```python
from build123d import *

# Parameters (mm, degrees)
EXTRUDE_1_DEPTH               = 10
SKETCH_2_R                    = 2.5
CUT_EXTRUDE_2_DEPTH           = 39.013155617
SKETCH_4_R                    = 4.5
CUT_EXTRUDE_3_DEPTH           = 2
CUT_EXTRUDE_3_DRAFT           = -45
CUT_EXTRUDE_3_PROFILE_2_DEPTH = 2
CUT_EXTRUDE_3_PROFILE_2_DRAFT = -45
CUT_EXTRUDE_3_PROFILE_3_DEPTH = 2
CUT_EXTRUDE_3_PROFILE_3_DRAFT = -45
CUT_EXTRUDE_3_PROFILE_4_DEPTH = 2
CUT_EXTRUDE_3_PROFILE_4_DRAFT = -45
SKETCH_5_R                    = 3
CUT_EXTRUDE_4_DEPTH           = 39.013155617


with BuildPart() as part:
    # Эскиз1 → Вытянуть1 (new body)
    with BuildSketch(Plane(origin=(0, 0, 0), x_dir=(0, 0, -1), z_dir=(1, 0, 0))):
        with BuildLine():
            Line((12.845232579, 11), (33, 11))
            Line((33, 11), (33, -11))
            Line((33, -11), (12.845232579, -11))
            ThreePointArc((12.845232579, -11), (11.757018204, -11.204326651), (10.817037961, -11.789473684))
            ThreePointArc((10.817037961, -11.789473684), (0, -16), (-10.817037961, -11.789473684))
            ThreePointArc((-10.817037961, -11.789473684), (-11.757018204, -11.204326651), (-12.845232579, -11))
            Line((-12.845232579, -11), (-33, -11))
            Line((-33, -11), (-33, 11))
            Line((-33, 11), (-12.845232579, 11))
            ThreePointArc((-12.845232579, 11), (-11.757018204, 11.204326651), (-10.817037961, 11.789473684))
            ThreePointArc((-10.817037961, 11.789473684), (0, 16), (10.817037961, 11.789473684))
            ThreePointArc((10.817037961, 11.789473684), (11.757018204, 11.204326651), (12.845232579, 11))
        make_face()
    extrude(amount=EXTRUDE_1_DEPTH)

    # Эскиз2 → Вытянуть2 (cut, through all)
    with BuildSketch(Plane(origin=(10, 0, 0), x_dir=(0, 0, -1), z_dir=(1, 0, 0))):
        with Locations((0, 10)):
            Circle(SKETCH_2_R)
        with Locations((10, 0)):
            Circle(SKETCH_2_R)
        with Locations((0, -10)):
            Circle(SKETCH_2_R)
        with Locations((-10, 0)):
            Circle(SKETCH_2_R)
    extrude(amount=-CUT_EXTRUDE_2_DEPTH, mode=Mode.SUBTRACT)


with BuildPart() as cut_extrude_3_tool:
    # Эскиз4 → Вытянуть3 (with draft: the straight prism first)
    with BuildSketch(Plane(origin=(10, 0, 0), x_dir=(0, 0, -1), z_dir=(1, 0, 0))):
        with Locations((0, 10)):
            Circle(SKETCH_4_R)
    extrude(amount=-CUT_EXTRUDE_3_DEPTH)
    # Вытянуть3: the draft: its side faces are tilted about the plane it starts from
    cut_extrude_3_sides = [cut_extrude_3_tool.faces().sort_by_distance(p)[0] for p in [
        (9, 10, 4.5),
    ]]
    draft(cut_extrude_3_sides, Plane(origin=(10, 0, 0), x_dir=(0, 0, -1), z_dir=(1, 0, 0)), CUT_EXTRUDE_3_DRAFT)


with BuildPart() as part_1:
    add(part.part)

    # Вытянуть3: cut by cut_extrude_3_tool
    add(cut_extrude_3_tool.part, mode=Mode.SUBTRACT)


with BuildPart() as cut_extrude_3_profile_2_tool:
    # Эскиз4 → Вытянуть3 profile 2 (with draft: the straight prism first)
    with BuildSketch(Plane(origin=(10, 0, 0), x_dir=(0, 0, -1), z_dir=(1, 0, 0))):
        with Locations((10, 0)):
            Circle(SKETCH_4_R)
    extrude(amount=-CUT_EXTRUDE_3_PROFILE_2_DEPTH)
    # Вытянуть3 profile 2: the draft: its side faces are tilted about the plane it starts from
    cut_extrude_3_profile_2_sides = [cut_extrude_3_profile_2_tool.faces().sort_by_distance(p)[0] for p in [
        (9, 0, -5.5),
    ]]
    draft(cut_extrude_3_profile_2_sides, Plane(origin=(10, 0, 0), x_dir=(0, 0, -1), z_dir=(1, 0, 0)), CUT_EXTRUDE_3_PROFILE_2_DRAFT)


with BuildPart() as part_2:
    add(part_1.part)

    # Вытянуть3 profile 2: cut by cut_extrude_3_profile_2_tool
    add(cut_extrude_3_profile_2_tool.part, mode=Mode.SUBTRACT)


with BuildPart() as cut_extrude_3_profile_3_tool:
    # Эскиз4 → Вытянуть3 profile 3 (with draft: the straight prism first)
    with BuildSketch(Plane(origin=(10, 0, 0), x_dir=(0, 0, -1), z_dir=(1, 0, 0))):
        with Locations((0, -10)):
            Circle(SKETCH_4_R)
    extrude(amount=-CUT_EXTRUDE_3_PROFILE_3_DEPTH)
    # Вытянуть3 profile 3: the draft: its side faces are tilted about the plane it starts from
    cut_extrude_3_profile_3_sides = [cut_extrude_3_profile_3_tool.faces().sort_by_distance(p)[0] for p in [
        (9, -10, 4.5),
    ]]
    draft(cut_extrude_3_profile_3_sides, Plane(origin=(10, 0, 0), x_dir=(0, 0, -1), z_dir=(1, 0, 0)), CUT_EXTRUDE_3_PROFILE_3_DRAFT)


with BuildPart() as part_3:
    add(part_2.part)

    # Вытянуть3 profile 3: cut by cut_extrude_3_profile_3_tool
    add(cut_extrude_3_profile_3_tool.part, mode=Mode.SUBTRACT)


with BuildPart() as cut_extrude_3_profile_4_tool:
    # Эскиз4 → Вытянуть3 profile 4 (with draft: the straight prism first)
    with BuildSketch(Plane(origin=(10, 0, 0), x_dir=(0, 0, -1), z_dir=(1, 0, 0))):
        with Locations((-10, 0)):
            Circle(SKETCH_4_R)
    extrude(amount=-CUT_EXTRUDE_3_PROFILE_4_DEPTH)
    # Вытянуть3 profile 4: the draft: its side faces are tilted about the plane it starts from
    cut_extrude_3_profile_4_sides = [cut_extrude_3_profile_4_tool.faces().sort_by_distance(p)[0] for p in [
        (9, 0, 14.5),
    ]]
    draft(cut_extrude_3_profile_4_sides, Plane(origin=(10, 0, 0), x_dir=(0, 0, -1), z_dir=(1, 0, 0)), CUT_EXTRUDE_3_PROFILE_4_DRAFT)


with BuildPart() as part_4:
    add(part_3.part)

    # Вытянуть3 profile 4: cut by cut_extrude_3_profile_4_tool
    add(cut_extrude_3_profile_4_tool.part, mode=Mode.SUBTRACT)

    # Эскиз5 → Вытянуть4 (cut, through all)
    with BuildSketch(Plane(origin=(10, 0, 0), x_dir=(0, 0, -1), z_dir=(1, 0, 0))):
        Circle(SKETCH_5_R)
    extrude(amount=-CUT_EXTRUDE_4_DEPTH, mode=Mode.SUBTRACT)


solid = part_4.part
```
Input: part model. Units: mm. Frame: model coordinates. A direction names the side the tool comes from. Coordinates: 2 decimals unless noted, no trailing zeros. Write each loop counter-clockwise with the first axis right and the second up, starting at its lowest first coordinate (ties: lowest second). Pieces come first, ordered by that corner, then holes. Notation, with made-up numbers: (-31, -9.75) - (23, -9.75) arc R7 cw to (23, -2.75) - close; hole circle Ø1 at (56.25, 82). An arc over 180 degrees is marked (long way). Put each result on its own line as item: value. Start each with the question number.
1) Contact query for flat-ended pins moving along their axis: pin 1 (3 mm diameter, centred on y = -10, z = 0, fed in from -X); pin 2 (6.5 mm diameter, centred on y = 0, z = 10, fed in from +X); pin 3 (1.5 mm diameter, centred on x = 8.5, y = 12, fed in from -Z). Output: stop coordinate, or through.
2) Reachability of faces 1 (the face through (5, -11, 23)), 2 (the face through (4.06, -12.44, 0.54)), 3 (the face through (5, 11, 23)), 4 (the face through (5, -11, -23)), 5 (the face through (10, -3.3, -0.5)) from +Z, -Z, +X, -X, +Y, -Y: full face, straight path, thin tool, end or side. Return the list, or none.
3) Ray query, L1, parallel to Y at x = 3.5, z = 10; L2, parallel to Y at x = 2.5, z = 2; L3, parallel to Y at x = 8, z = -19.5. Return the intervals inside material, ascending.
4) Cut plane A-A (y = 0). Return the cut outline in (x, z).
5) Cut plane B-B (z = 10). Return the cut outline in (x, y).
6) Cut plane D-D (x = 8.75). Return the cut outline in (y, z).
7) Cut plane C-C (y = 10). Return the cut outline in (x, z).
8) Mould query, pull axis Y, two halves, no side actions, for faces 6 (the face through (5, 16, 0)), 7 (the face through (0, 4, 0)), 8 (the face through (8.125, -11.597, 2.083)). Classes: pulls with the +Y half, pulls with the -Y half, needs draft (parallel to the pull), parting line crosses it, or undercut.
Resolved:
1. pin 1: passes through
1. pin 2: stops at x = 8.75
1. pin 3: stops at z = -11.65
2. face 1: +Z, +X, -X, -Y
2. face 2: +X, -X
2. face 3: +Z, +X, -X, +Y
2. face 4: -Z, +X, -X, -Y
2. face 5: +Z, -Z, +X, +Y, -Y
3. L1: y = -12.49 to -2.5, 2.5 to 12.49
3. L2: y = -15.87 to -11.5, -8.5 to -2.24, 2.24 to 8.5, 11.5 to 15.87
3. L3: y = -11 to 11
4. outline: (0, -33) - (10, -33) - (10, -14.5) - (8, -12.5) - (0, -12.5) - close; (0, -7.5) - (8, -7.5) - (10, -5.5) - (10, -3) - (0, -3) - close; (0, 3) - (10, 3) - (10, 5.5) - (8, 7.5) - (0, 7.5) - close; (0, 12.5) - (8, 12.5) - (10, 14.5) - (10, 33) - (0, 33) - close
5. outline: (0, -12.49) - (10, -12.49) - (10, -4.5) - (8, -2.5) - (0, -2.5) - close; (0, 2.5) - (8, 2.5) - (10, 4.5) - (10, 12.49) - (0, 12.49) - close
6. outline: (-11.79, -10.82) arc R3 cw to (-11, -12.85) - (-11, -33) - (11, -33) - (11, -12.85) arc R3 cw to (11.79, -10.82) arc R16 ccw to (11.79, 10.82) arc R3 cw to (11, 12.85) - (11, 33) - (-11, 33) - (-11, 12.85) arc R3 cw to (-11.79, 10.82) arc R16 ccw to start; hole circle Ø6.5 at (-10, 0); hole circle Ø6.5 at (0, -10); hole circle Ø6.5 at (0, 10); hole circle Ø6 at (0, 0); hole circle Ø6.5 at (10, 0)
7. outline: (0, -33) - (10, -33) - (10, -4.5) - (8, -2.5) - (0, -2.5) - close; (0, 2.5) - (8, 2.5) - (10, 4.5) - (10, 33) - (0, 33) - close
8. face 6: pulls with the +Y half
8. face 7: needs draft
8. face 8: undercut
